Work out the finished part from the listing and answer in its coordinate system (mm). Face numbers are marked on the shaded views. A direction names the side the tool comes from. Coordinates: 2 decimals unless noted, no trailing zeros. Order: outer loops, then holes, each group sorted by start corner. A loop starts at its lowest first (then second) coordinate and runs counter-clockwise, first axis right, second up.
1. The part is cut by section C-C, the plane y = 0. Give the vertices of the cut face in (x, z), then the cut area to 3 significant figures.
2. A tool of negligible diameter and unlimited length cuts with its end or side. For the marked faces 1, 2 and 3, from which of +Z, -Z, +X, -X, +Y, -Y can it reach the whole face along a straight path? Write none if from no direction.
3. Flat-ended cylindrical pins translate along their axes: pin 1 Ø12 at (x, y) = (5.5, 1.5) entering from -Z; pin 2 Ø5 at (x, y) = (6, 1) entering from +Z; pin 3 Ø10 at (x, z) = (4.5, 20) entering from +Y; pin 4 Ø6 at (x, z) = (0, 21) entering from -Y. Find the tip coordinate at first contact, or state that the pin passes through.
4. The part is cut by section B-B, the plane z = 2. Give the vertices of the cut face in (x, y).
5. Find the intervals of material crossed by probe 1 along Y at (x, z) = (0, 2.5); probe 2 along Z at (x, y) = (-7, 1.75); probe 3 along X at (y, z) = (3, 3), in increasing order.
6. The part is cut by section A-A, the plane x = 0. Give the vertices of the cut face in (y, z).
7. The part is cut by section D-D, the plane y = 10. Give the vertices of the cut face in (x, z).
8. Determine the mould class of the marked faces 4, 5, 6 and 7 for opening direction X: +X half, -X half, draft (parallel to the pull), parting line (faces both ways), or undercut.
```python
from build123d import *

# Parameters (mm, degrees)
SKETCH_1_R             = 2.5
SKETCH_1_R_2           = 1
EXTRUDE_2_DEPTH        = 24
EXTRUDE_3_DEPTH        = 2
EXTRUDE_3_DEPTH_BACK   = 1
SKETCH_3_R             = 1.5
EXTRUDE_3_2_DEPTH      = 2
EXTRUDE_3_2_DEPTH_BACK = 1
EXTRUDE_3_3_DEPTH      = 2
EXTRUDE_3_3_DEPTH_BACK = 1
SKETCH_4_R             = 2.23
CUT_EXTRUDE_1_DEPTH    = 2
EXTRUDE_6_DEPTH        = 3
EXTRUDE_6_DEPTH_BACK   = 0.5
SKETCH_10_R            = 2.35
SKETCH_10_R_2          = 2.23
CUT_EXTRUDE_2_DEPTH    = 1
SKETCH_11_R            = 3.7
CUT_EXTRUDE_3_DEPTH    = 2
SKETCH_12_R            = 1
CUT_EXTRUDE_4_DEPTH    = 27.532998323
FILLET_5_R             = 1
FILLET_6_R             = 4
SKETCH_14_R            = 2.75
SKETCH_14_R_2          = 2.23
CUT_EXTRUDE_5_DEPTH    = 2


with BuildPart() as part:
    # Sketch 1 → Extrude 2 (new body)
    with BuildSketch(Plane.XY):
        Circle(SKETCH_1_R)
        Circle(SKETCH_1_R_2, mode=Mode.SUBTRACT)
    extrude(amount=EXTRUDE_2_DEPTH)

    # Sketch 4 → Cut-Extrude 1 (cut)
    with BuildSketch(Plane(origin=(0, 0, 0), x_dir=(-1, 0, 0), z_dir=(0, 0, -1))):
        Circle(SKETCH_4_R)
    extrude(amount=-CUT_EXTRUDE_1_DEPTH, mode=Mode.SUBTRACT)



with BuildPart() as body_2:
    # Sketch 3 → Extrude 3 (new, two sides: drawn at the far end of the back side and taken through both)
    with BuildSketch(Plane.XY.offset(-EXTRUDE_3_DEPTH_BACK)):
        with Locations((0, 10)):
            Circle(SKETCH_3_R)
    extrude(amount=EXTRUDE_3_DEPTH + EXTRUDE_3_DEPTH_BACK)


with BuildPart() as body_3:
    # Sketch 3 → Extrude 3 2 (new, two sides: drawn at the far end of the back side and taken through both)
    with BuildSketch(Plane.XY.offset(-EXTRUDE_3_2_DEPTH_BACK)):
        with Locations((8.660254038, -5)):
            Circle(SKETCH_3_R)
    extrude(amount=EXTRUDE_3_2_DEPTH + EXTRUDE_3_2_DEPTH_BACK)


with BuildPart() as body_4:
    # Sketch 3 → Extrude 3 3 (new, two sides: drawn at the far end of the back side and taken through both)
    with BuildSketch(Plane.XY.offset(-EXTRUDE_3_3_DEPTH_BACK)):
        with Locations((-8.660254038, -5)):
            Circle(SKETCH_3_R)
    extrude(amount=EXTRUDE_3_3_DEPTH + EXTRUDE_3_3_DEPTH_BACK)


with BuildPart() as part_1:
    add(part.part)

    add(body_2.part)  # Extrude 6 merges body 2

    add(body_3.part)  # Extrude 6 merges body 3

    add(body_4.part)  # Extrude 6 merges body 4
    # Sketch 5 → Extrude 6 (add, two sides: drawn at the far end of the back side and taken through both)
    with BuildSketch(Plane.XY.offset(2).offset(-EXTRUDE_6_DEPTH_BACK)):
        Polygon((0, 14), (-12.124355653, -7), (12.124355653, -7), align=None)
    extrude(amount=EXTRUDE_6_DEPTH + EXTRUDE_6_DEPTH_BACK)

    # Sketch 10 → Cut-Extrude 2 (cut)
    with BuildSketch(Plane(origin=(0, 0, 0), x_dir=(-1, 0, 0), z_dir=(0, 0, -1))):
        Circle(SKETCH_10_R)
        Circle(SKETCH_10_R_2, mode=Mode.SUBTRACT)
    extrude(amount=-CUT_EXTRUDE_2_DEPTH, mode=Mode.SUBTRACT)

    # Sketch 11 → Cut-Extrude 3 (cut)
    with BuildSketch(Plane(origin=(0, 0, 1.5), x_dir=(-1, 0, 0), z_dir=(0, 0, -1))):
        Circle(SKETCH_11_R)
    extrude(amount=-CUT_EXTRUDE_3_DEPTH, mode=Mode.SUBTRACT)


with BuildPart() as cut_extrude_3_piece_1:
    # of the separate pieces the step leaves, piece 1, a body of its own (cut_extrude_3_pieces)
    add(part_1.part.solids().sort_by_distance((0, 14, 1.5))[0])

    # Sketch 12 → Cut-Extrude 4 (cut, through all)
    with BuildSketch(Plane.XY.offset(5)):
        with Locations(Location((0, 0, 0), (0, 0, 180))):
            Circle(SKETCH_12_R)
    extrude(amount=-CUT_EXTRUDE_4_DEPTH, mode=Mode.SUBTRACT)

    # Fillet 5
    fillet_5_edges = [cut_extrude_3_piece_1.edges().sort_by_distance(p)[0] for p in [
        (0, 14, 3.25),
        (12.124355653, -7, 3.25),
        (-12.124355653, -7, 3.25),
    ]]
    fillet(fillet_5_edges, radius=FILLET_5_R)

    # Fillet 6
    fillet_6_edges = [cut_extrude_3_piece_1.edges().sort_by_distance(p)[0] for p in [
        (-2.5, 0, 5),
    ]]
    fillet(fillet_6_edges, radius=FILLET_6_R)


with BuildPart() as cut_extrude_3_piece_2:
    # of the separate pieces the step leaves, piece 2, a body of its own (cut_extrude_3_pieces)
    add(part_1.part.solids().sort_by_distance((2.5, 0, 0))[0])

    # Sketch 14 → Cut-Extrude 5 (cut)
    with BuildSketch(Plane(origin=(0, 0, 0), x_dir=(-1, 0, 0), z_dir=(0, 0, -1))):
        Circle(SKETCH_14_R)
        Circle(SKETCH_14_R_2, mode=Mode.SUBTRACT)
    extrude(amount=-CUT_EXTRUDE_5_DEPTH, mode=Mode.SUBTRACT)


solid = cut_extrude_3_piece_1.part
```
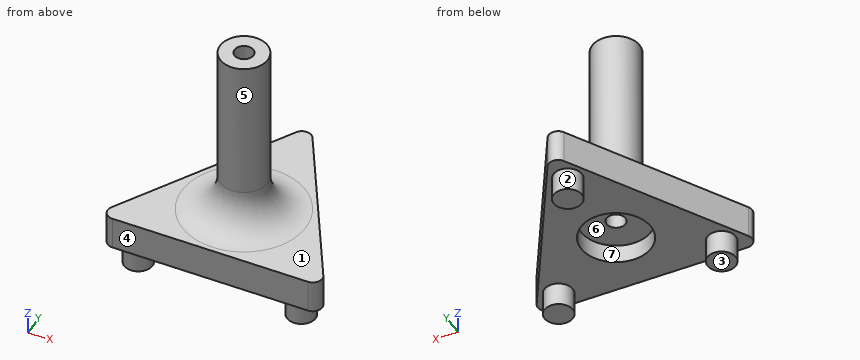
Geometry says:
1. outline: (-8.08, 1.5) - (-3.7, 1.5) - (-3.7, 3.5) - (-1, 3.5) - (-1, 24) - (-2.5, 24) - (-2.5, 9) arc R4 cw to (-6.5, 5) - (-8.08, 5) - close; (1, 3.5) - (3.7, 3.5) - (3.7, 1.5) - (8.08, 1.5) - (8.08, 5) - (6.5, 5) arc R4 cw to (2.5, 9) - (2.5, 24) - (1, 24) - close
1. area: 103 mm2
2. face 1: +Z
2. face 2: -Z
2. face 3: -Z, +X, -X, +Y, -Y
3. pin 1: stops at z = -1
3. pin 2: stops at z = 6.26
3. pin 3: stops at y = 2.5
3. pin 4: stops at y = -2.5
4. outline: (-11.26, -5.5) arc R1 ccw to (-10.39, -7) - (10.39, -7) arc R1 ccw to (11.26, -5.5) - (0.87, 12.5) arc R1 ccw to (-0.87, 12.5) - close; hole circle Ø7.4 at (0, 0)
5. probe 1: y = -7 to -3.7, 3.7 to 13
5. probe 2: z = 1.5 to 5
5. probe 3: x = -6.35 to -2.17, 2.17 to 6.35
6. outline: (-7, 1.5) - (-3.7, 1.5) - (-3.7, 3.5) - (-1, 3.5) - (-1, 24) - (-2.5, 24) - (-2.5, 9) arc R4 cw to (-6.5, 5) - (-7, 5) - close; (1, 3.5) - (3.7, 3.5) - (3.7, 1.5) - (8.5, 1.5) - (8.5, -1) - (11.5, -1) - (11.5, 1.5) - (13, 1.5) - (13, 5) - (6.5, 5) arc R4 cw to (2.5, 9) - (2.5, 24) - (1, 24) - close
7. outline: (-2.31, 1.5) - (-1.5, 1.5) - (-1.5, -1) - (1.5, -1) - (1.5, 1.5) - (2.31, 1.5) - (2.31, 5) - (-2.31, 5) - close
8. face 4: draft
8. face 5: parting line
8. face 6: undercut
8. face 7: undercut
